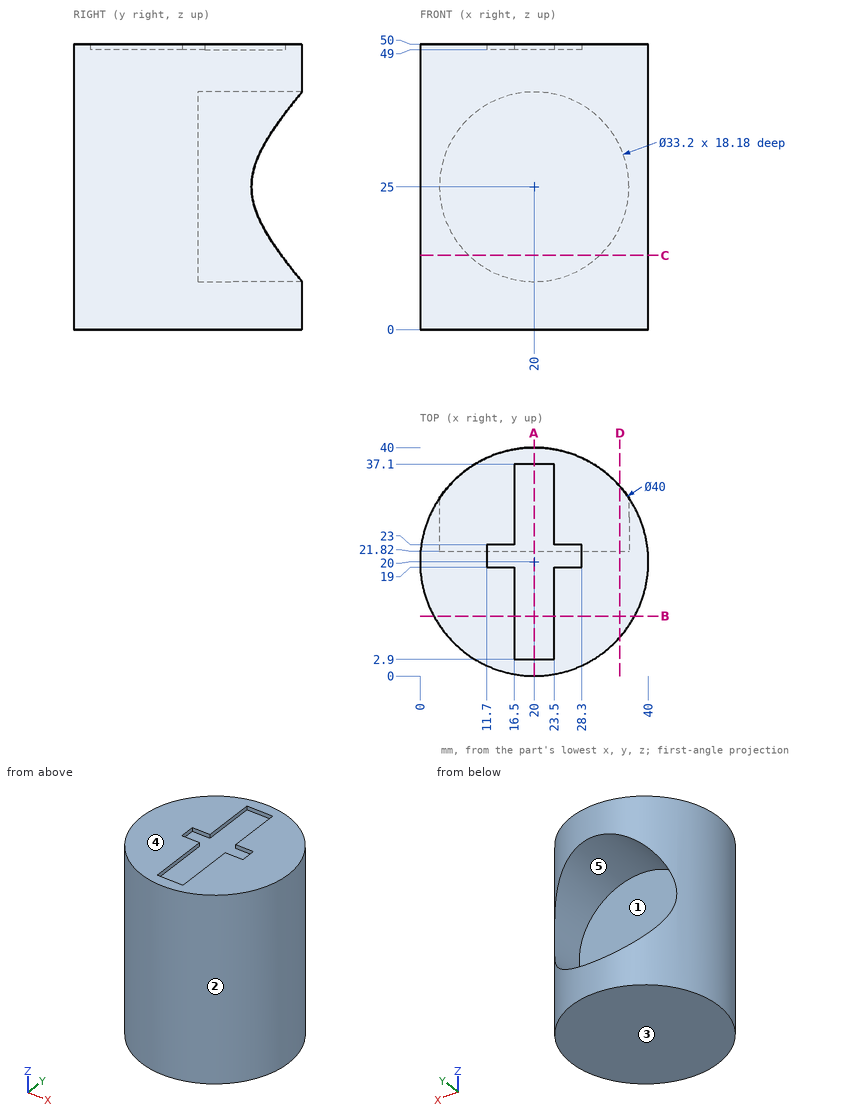
Print and shaded views of the part. All mm, measured from the part's lowest x, y and z. A direction names the side the tool comes from. Round coordinates to 2 decimals unless told otherwise and drop trailing zeros. Write each loop counter-clockwise with the first axis right and the second up, starting at its lowest first coordinate (ties: lowest second). Pieces come first, ordered by that corner, then holes. Notation, with made-up numbers: (28.25, 22.5) - (58.25, 22.5) arc R15 ccw to (58.25, 31.5) - close; hole circle Ø10 at (81.5, 51.5). An arc over 180 degrees is marked (long way). Write each question's results on one line, items separated by ' | '. Start each with the question number.
Item 1: Which spindle directions (+Z, -Z, +X, -X, +Y, -Y) get a long thin tool onto all of the face, cutting with end or side? Do the marked faces 4 and 5. Say none if no direction does.
Item 2: Saw through at C-C (z = 13). Write the cut outline in (x, y).
Item 3: Mould opens along X. For the marked faces 1, 2 and 3 say: pulls with the +X half, pulls with the -X half, needs draft (parallel to the pull), parting line crosses it, or undercut.
Item 4: Wall check: L1, parallel to X at y = 19.5, z = 43.5; L2, parallel to X at y = 27.25, z = 25; L3, parallel to Z at x = 30.5, y = 34. Give the ranges that are in metal, low to high. Write a range as [from, to].
Item 5: Saw through at B-B (y = 10.5). Write the cut outline in (x, z).
Item 6: Saw through at A-A (x = 20). Write the cut outline in (y, z).
Item 7: Drop flat-ended pins along their axis: P1, Ø0.5, axis at y = 21, z = 49.5, coming from the +X side; P2, Ø4, axis at x = 4, z = 37, coming from the -Y side; P3, Ø1.5, axis at y = 21.5, z = 25, coming from the -X side. Give the stop position or say it passes through.
Item 8: Saw through at D-D (x = 35). Write the cut outline in (y, z).
Results are:
1) face 4: +Z, +X, -X, +Y, -Y | face 5: +Y
2) outline: (8.53, 21.82) - (8.53, 36.38) arc R20 ccw (long way) to (31.47, 36.38) - (31.47, 21.82) - close
3) face 1: undercut | face 2: parting line crosses it | face 3: needs draft
4) L1: x = [0.01, 39.99] | L2: x = [1.36, 3.4], [36.6, 38.64] | L3: z = [0, 12.14], [37.86, 50]
5) outline: (2.4, 0) - (37.6, 0) - (37.6, 50) - (23.5, 50) - (23.5, 49) - (16.5, 49) - (16.5, 50) - (2.4, 50) - close
6) outline: (0, 0) - (40, 0) - (40, 8.4) - (21.82, 8.4) - (21.82, 41.6) - (40, 41.6) - (40, 50) - (37.1, 50) - (37.1, 49) - (2.9, 49) - (2.9, 50) - (0, 50) - close
7) P1: stops at x = 39.99 | P2: stops at y = 5.72 | P3: stops at x = 0.01
8) outline: (6.77, 0) - (33.23, 0) - (33.23, 17.89) - (21.82, 17.89) - (21.82, 32.11) - (33.23, 32.11) - (33.23, 50) - (6.77, 50) - close
